Input: part model. Units: mm. Frame: model coordinates. A direction names the side the tool comes from. Coordinates: 2 decimals unless noted, no trailing zeros. Loops run counter-clockwise (first coordinate to the right, second up) from the corner with the lowest first, then second, coordinate; pieces in that order, holes last. Notation, with made-up numbers: M 14.25,-12 L 23.25,-12 A27 ccw 23.25,10 Z; hole C -17.5,-2 d10. An arc over 180 degrees is marked long. Use a Markdown table: item, result. Add a question column.
1. Draft query along Y for faces 3 (the flat face through (-20, 1, 4)), 4 (the flat face through (-9, -33.7, 4)), 5 (the flat face through (-9, 40, 4)). Return one class per face: +Y half, -Y half, draft (parallel to the pull), parting line (faces both ways), or undercut.
2. Line query: L1, parallel to Z at x = 0, y = 36.5; L2, parallel to Y at x = 7, z = 92.5; L3, parallel to X at y = 3, z = -260. Output: solid intervals per line, ascending. Write a range as [from, to].
3. Section A-A on z = 155. Output: boundary loops of the cut face in (x, y), then the cut area to 3 significant figures.
4. Set-up query: faces 1 (the cylindrical face through (7.493, 36.806, 4.67)), 2 (the flat face through (-13.7, 0, 4)). Return all of +Z, -Z, +X, -X, +Y, -Y with unobstructed straight access to the full face (end or side cutting, diameter ignored); none if empty.
5. Section B-B on x = 0. Output: boundary loops of the cut face in (y, z), then the cut area to 3 significant figures.
6. Section D-D on z = -167. Output: boundary loops of the cut face in (x, y).
7. Section C-C on y = -10. Output: boundary loops of the cut face in (x, z), then the cut area to 3 significant figures.
```python
from build123d import *

# Parameters (mm, degrees)
SKETCH1_W             = 40
SKETCH1_H             = 80
SKETCH1_W_2           = 27.4
SKETCH1_H_2           = 67.4
M12_CLEARANCE_HOLE1_D = 15


with BuildPart() as part:
    # Sweep1: sweep along a curve in space
    with BuildLine() as sweep1_path:
        add(Edge.make_bspline(
            [(0, 0, -300), (0, 0, 300)],
            knots=[0, 0, 1, 1], degree=1))
    # Sketch1 → Sweep1 (sweep)
    with BuildSketch(Plane.XY):
        Rectangle(SKETCH1_W, SKETCH1_H)
        Rectangle(SKETCH1_W_2, SKETCH1_H_2, mode=Mode.SUBTRACT)
    sweep(path=sweep1_path.line)

    # M12 Clearance Hole1 (through all)
    with Locations(Plane(origin=(0, 40, 0), x_dir=(1, 0, 0), z_dir=(0, 1, 0))):
        with Locations((0, -155), (0, -5)):
            Hole(M12_CLEARANCE_HOLE1_D / 2)


solid = part.part
```
Answers below:
| question | item | result |
|---|---|---|
| 1 | face 3 | draft |
| 1 | face 4 | undercut |
| 1 | face 5 | +Y half |
| 2 | L1 | z = [-300, -2.5], [12.5, 147.5], [162.5, 300] |
| 2 | L2 | y = [-40, -33.7], [33.7, 40] |
| 2 | L3 | x = [-20, -13.7], [13.7, 20] |
| 3 | outline | M -20,-40 L -7.5,-40 L -7.5,-33.7 L -13.7,-33.7 L -13.7,33.7 L -7.5,33.7 L -7.5,40 L -20,40 Z; M 7.5,-40 L 20,-40 L 20,40 L 7.5,40 L 7.5,33.7 L 13.7,33.7 L 13.7,-33.7 L 7.5,-33.7 Z |
| 3 | area | 1,160 mm² |
| 4 | face 1 | +Y, -Y |
| 4 | face 2 | +Z, -Z |
| 5 | outline | M -40,-300 L -33.7,-300 L -33.7,-2.5 L -40,-2.5 Z; M -40,12.5 L -33.7,12.5 L -33.7,147.5 L -40,147.5 Z; M -40,162.5 L -33.7,162.5 L -33.7,300 L -40,300 Z; M 33.7,-300 L 40,-300 L 40,-2.5 L 33.7,-2.5 Z; M 33.7,12.5 L 40,12.5 L 40,147.5 L 33.7,147.5 Z; M 33.7,162.5 L 40,162.5 L 40,300 L 33.7,300 Z |
| 5 | area | 7,180 mm² |
| 6 | outline | M -20,-40 L 20,-40 L 20,40 L -20,40 Z; hole M -13.7,-33.7 L 13.7,-33.7 L 13.7,33.7 L -13.7,33.7 Z |
| 7 | outline | M -20,-300 L -13.7,-300 L -13.7,300 L -20,300 Z; M 13.7,-300 L 20,-300 L 20,300 L 13.7,300 Z |
| 7 | area | 7,560 mm² |
